The model under review builds one solid part; all positions refer to its coordinate system, in mm. Face numbers are marked on the shaded views. A direction names the side the tool comes from. Round coordinates to 2 decimals unless told otherwise and drop trailing zeros. Write each loop counter-clockwise with the first axis right and the second up, starting at its lowest first coordinate (ties: lowest second). Pieces come first, ordered by that corner, then holes.
Item 1: Machinability: for the marked faces 4 and 5, which of the approach directions +Z, -Z, +X, -X, +Y, -Y give a long, thin tool a straight path to every point of the face, cutting with its end or side? Answer none if there is none.
Item 2: Draft analysis for pull direction Y (two halves, no side actions). For the marked faces 1, 2 and 3, state which applies: +Y half, -Y half, draft (parallel to the pull), parting line (faces both ways), or undercut.
Item 3: Add section B-B (x = 0). Give the boundary of the cut face in (y, z) (3 decimals), plus the area to 3 significant figures.
Item 4: Clearance check with flat-ended pins moving along their axes: pin 1 Ø6 at (y, z) = (5, 18.5) entering from -X; pin 2 Ø3 at (x, z) = (19, 11) entering from +Y; pin 3 Ø2 at (x, z) = (-1, 16) entering from -Y (3 decimals). State where each tip first meets the part, or that it passes through.
Item 5: To check wall thickness, follow L1, parallel to Y at x = 0, z = 21.5 (3 decimals); L2, parallel to X at y = 0.5, z = 4.75; L3, parallel to Z at x = -9.5, y = 8.5. State the ranges of each line that lie inside material, in increasing order.
Item 6: Add section C-C (y = 0). Give the boundary of the cut face in (x, z).
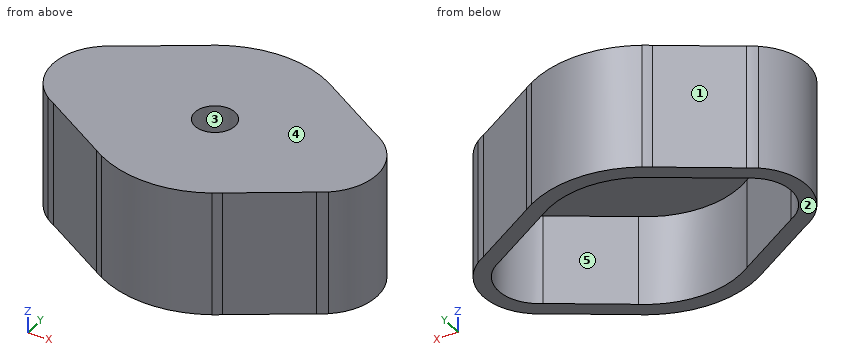
```python
from build123d import *

# Parameters (mm, degrees)
F1_DEPTH = 25
F3_DEPTH = 18
F4_R     = 4
F5_DEPTH = 25.001


with BuildPart() as f1:
    # F0 (on Top) → F1 (new body)
    with BuildSketch(Plane.XY):
        with BuildLine():
            Line((-10.875151469, -19.2677633763), (-12.3969796785, -18.3256792466))
            ThreePointArc((-12.3969796785, -18.3256792466), (-11.6455958484, -18.8121163705), (-10.875151469, -19.2677633763))
        make_face()
        with BuildLine():
            Line((-25.9545587129, -9.9328922254), (-12.3969796785, -18.3256792466))
            Line((-12.3969796785, -18.3256792466), (-10.875151469, -19.2677633763))
            ThreePointArc((-10.875151469, -19.2677633763), (0, -22.125), (10.875151469, -19.2677633763))
            Line((10.875151469, -19.2677633763), (12.3969796785, -18.3256792466))
            Line((12.3969796785, -18.3256792466), (25.9545587129, -9.9328922254))
            Line((25.9545587129, -9.9328922254), (27.6815068609, -8.8638290861))
            ThreePointArc((27.6815068609, -8.8638290861), (32.1, 0), (27.6815068609, 8.8638290861))
            Line((27.6815068609, 8.8638290861), (25.9545587129, 9.9328922254))
            Line((25.9545587129, 9.9328922254), (12.3969796785, 18.3256792466))
            Line((12.3969796785, 18.3256792466), (10.875151469, 19.2677633763))
            ThreePointArc((10.875151469, 19.2677633763), (0, 22.125), (-10.875151469, 19.2677633763))
            Line((-10.875151469, 19.2677633763), (-12.3969796785, 18.3256792466))
            Line((-12.3969796785, 18.3256792466), (-25.9545587129, 9.9328922254))
            Line((-25.9545587129, 9.9328922254), (-27.6815068609, 8.8638290861))
            ThreePointArc((-27.6815068609, 8.8638290861), (-32.1, 0), (-27.6815068609, -8.8638290861))
            Line((-27.6815068609, -8.8638290861), (-25.9545587129, -9.9328922254))
        make_face()
        with BuildLine():
            ThreePointArc((-25.9545587129, 9.9328922254), (-26.8425362222, 9.4379431282), (-27.6815068609, 8.8638290861))
            Line((-27.6815068609, 8.8638290861), (-25.9545587129, 9.9328922254))
        make_face()
        with BuildLine():
            ThreePointArc((-10.875151469, 19.2677633763), (-11.6455958484, 18.8121163705), (-12.3969796785, 18.3256792466))
            Line((-12.3969796785, 18.3256792466), (-10.875151469, 19.2677633763))
        make_face()
        with BuildLine():
            ThreePointArc((12.3969796785, 18.3256792466), (11.6455958484, 18.8121163705), (10.875151469, 19.2677633763))
            Line((10.875151469, 19.2677633763), (12.3969796785, 18.3256792466))
        make_face()
        with BuildLine():
            Line((25.9545587129, 9.9328922254), (27.6815068609, 8.8638290861))
            ThreePointArc((27.6815068609, 8.8638290861), (26.8425362222, 9.4379431282), (25.9545587129, 9.9328922254))
        make_face()
        with BuildLine():
            Line((27.6815068609, -8.8638290861), (25.9545587129, -9.9328922254))
            ThreePointArc((25.9545587129, -9.9328922254), (26.8425362222, -9.4379431282), (27.6815068609, -8.8638290861))
        make_face()
        with BuildLine():
            ThreePointArc((-27.6815068609, -8.8638290861), (-26.8425362222, -9.4379431282), (-25.9545587129, -9.9328922254))
            Line((-25.9545587129, -9.9328922254), (-27.6815068609, -8.8638290861))
        make_face()
        with BuildLine():
            Line((12.3969796785, -18.3256792466), (10.875151469, -19.2677633763))
            ThreePointArc((10.875151469, -19.2677633763), (11.6455958484, -18.8121163705), (12.3969796785, -18.3256792466))
        make_face()
    extrude(amount=F1_DEPTH)

    # F2 (on Top) → F3 (cut)
    with BuildSketch(Plane.XY):
        with BuildLine():
            ThreePointArc((-24.4535832454, 7.2161457692), (-28.9999998122, 0), (-24.4535832454, -7.2161457692))
            Line((-24.4535832454, -7.2161457692), (-10.7099389872, -15.7241160243))
            ThreePointArc((-10.7099389872, -15.7241160243), (0, -19.0249998122), (10.7099389872, -15.7241160243))
            Line((10.7099389872, -15.7241160243), (24.4535832454, -7.2161457692))
            ThreePointArc((24.4535832454, -7.2161457692), (28.9999998122, 0), (24.4535832454, 7.2161457692))
            Line((24.4535832454, 7.2161457692), (10.7099389872, 15.7241160243))
            ThreePointArc((10.7099389872, 15.7241160243), (0, 19.0249998122), (-10.7099389872, 15.7241160243))
            Line((-10.7099389872, 15.7241160243), (-24.4535832454, 7.2161457692))
        make_face()
    extrude(amount=F3_DEPTH, mode=Mode.SUBTRACT)

    # F4 (on Top) → F5 (cut, through all)
    with BuildSketch(Plane.XY):
        Circle(F4_R)
    extrude(amount=F5_DEPTH, mode=Mode.SUBTRACT)


solid = f1.part
```
Numbers:
1. face 4: +Z, +X, -X, +Y, -Y
1. face 5: -Z
2. face 1: +Y half
2. face 2: draft
2. face 3: undercut
3. outline: (-22.125, 0) - (-19.025, 0) - (-19.025, 18) - (-4, 18) - (-4, 25) - (-22.125, 25) - close; (4, 18) - (19.025, 18) - (19.025, 0) - (22.125, 0) - (22.125, 25) - (4, 25) - close
3. area: 365 mm2
4. pin 1: stops at x = -31.92
4. pin 2: stops at y = 15.17
4. pin 3: stops at y = -22.125
5. L1: y = -22.125 to -4, 4 to 22.125
5. L2: x = -32.09 to -28.98, 28.98 to 32.09
5. L3: z = 18 to 25
6. outline: (-32.1, 0) - (-29, 0) - (-29, 18) - (-4, 18) - (-4, 25) - (-32.1, 25) - close; (4, 18) - (29, 18) - (29, 0) - (32.1, 0) - (32.1, 25) - (4, 25) - close
